from build123d import *

# Parameters (mm, degrees)
BOSS_EXTRUDE2_DEPTH = 2
SKETCH2_R           = 0.8
CUT_EXTRUDE1_DEPTH  = 2
FILLET1_R           = 2


with BuildPart() as part:
    # Sketch1 → Boss-Extrude2 (new body)
    with BuildSketch(Plane.XY):
        Polygon((17, 10.5), (17, 10), (34, 10), (34, 20), (17, 20), (17, 14.5), (27, 14.5), (27, 10.5), align=None)
        Polygon((34, 10), (17, 10), (17, 9.5), (27, 9.5), (27, 5.5), (17, 5.5), (17, 0), (34, 0), align=None)
        Polygon((17, 10), (0, 10), (0, 0), (17, 0), (17, 5.5), (7, 5.5), (7, 9.5), (17, 9.5), align=None)
        Polygon((0, 20), (0, 10), (17, 10), (17, 10.5), (7, 10.5), (7, 14.5), (17, 14.5), (17, 20), align=None)
    extrude(amount=BOSS_EXTRUDE2_DEPTH)

    # Sketch2 → Cut-Extrude1 (cut)
    with BuildSketch(Plane.XY.offset(2)):
        with Locations((2, 2)):
            Circle(SKETCH2_R)
        with Locations((2, 18)):
            Circle(SKETCH2_R)
        with Locations((32, 18)):
            Circle(SKETCH2_R)
        with Locations((32, 2)):
            Circle(SKETCH2_R)
    extrude(amount=-CUT_EXTRUDE1_DEPTH, mode=Mode.SUBTRACT)

    # Fillet1
    fillet1_edges = [part.edges().sort_by_distance(p)[0] for p in [
        (7, 9.5, 1),
        (7, 5.5, 1),
        (27, 9.5, 1),
        (27, 5.5, 1),
        (27, 10.5, 1),
        (27, 14.5, 1),
        (7, 10.5, 1),
        (7, 14.5, 1),
    ]]
    fillet(fillet1_edges, radius=FILLET1_R - 0.0001)  # a hair under: the kernel refuses the full size


solid = part.part
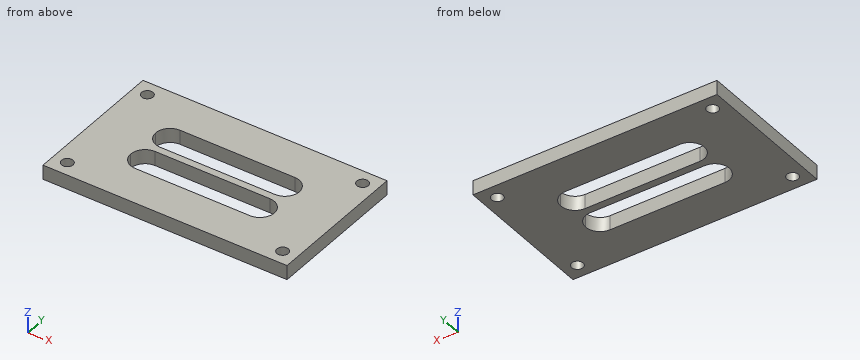
Input: part model. Units: mm. Frame: model coordinates. Coordinates: 2 decimals unless noted, no trailing zeros. Order: outer loops, then holes, each group sorted by start corner. A loop starts at its lowest first (then second) coordinate and runs counter-clockwise, first axis right, second up. Notation, with made-up numbers: M 52.25,20 L 102.25,20 A26 cw 102.25,40 Z; hole C 24,18.25 d2. An arc over 180 degrees is marked long. Answer as CSV lines item,"result".
1. Section A-A (y = 18). Return the cut outline in (x, z).
Reported:
outline,"M 0,0 L 1.2,0 L 1.2,2 L 0,2 Z; M 2.8,0 L 31.2,0 L 31.2,2 L 2.8,2 Z; M 32.8,0 L 34,0 L 34,2 L 32.8,2 Z"
2. Material intervals for line 1 (Y direction, x = 2, z = 1.55); line 2 (Y direction, x = 20.5, z = 1.65); line 3 (X direction, y = 2.5, z = 1.6), sorted ascending. Write a range as from..to.
Reported:
line 1,"0..1.2, 2.8..17.2, 18.8..20"
line 2,"0..5.5, 9.5..10.5, 14.5..20"
line 3,"0..1.38, 2.62..31.38, 32.62..34"
3. Section B-B (x = 2). Return the cut outline in (y, z), then the cut area to 3 significant figures.
Reported:
outline,"M 0,0 L 1.2,0 L 1.2,2 L 0,2 Z; M 2.8,0 L 17.2,0 L 17.2,2 L 2.8,2 Z; M 18.8,0 L 20,0 L 20,2 L 18.8,2 Z"
area,"33.6 mm2"
4. Section C-C (z = 1.2). State how many separate pieces and enclosed holes the cut face has, then the cut area to 3 significant figures.
Reported:
separate pieces,"1"
enclosed holes,"6"
area,"519 mm2"
5. Section D-D (y = 6.5). Return the cut outline in (x, z).
Reported:
outline,"M 0,0 L 7.27,0 L 7.27,2 L 0,2 Z; M 26.73,0 L 34,0 L 34,2 L 26.73,2 Z"
6. First-contact query: P1, Ø1.3, axis at x = 32, y = 2, coming from the +Z side. Flat tip, straight axial feed; report the tip coordinate or a pass-through.
Reported:
P1,"through"
